```python
from build123d import *

# Parameters (mm, degrees)
SKETCH1_R           = 2.5
BOSS_EXTRUDE1_DEPTH = 4
SKETCH2_R           = 5
BOSS_EXTRUDE2_DEPTH = 0.75
M1_6_NUT_DEPTH      = 9.124038405
M1_6_NUT_DEPTH_BACK = 9.124038405
SKETCH5_W           = 6.5
SKETCH5_H           = 0.25
CUT_EXTRUDE1_DEPTH  = 9.124038405


with BuildPart() as part:
    # Sketch1 → Boss-Extrude1 (new, symmetric)
    with BuildSketch(Plane(origin=(0, 0, 0), x_dir=(0, 0, -1), z_dir=(1, 0, 0))):
        Circle(SKETCH1_R)
    extrude(amount=BOSS_EXTRUDE1_DEPTH, both=True)

    # Sketch2 → Boss-Extrude2 (add)
    with BuildSketch(Plane(origin=(4, 0, 0), x_dir=(0, 0, -1), z_dir=(1, 0, 0))):
        Circle(SKETCH2_R)
    boss_extrude2 = extrude(amount=-BOSS_EXTRUDE2_DEPTH)

    # Mirror1: Boss-Extrude2 across plane
    add(boss_extrude2.mirror(Plane(origin=(0, 0, 0), x_dir=(0, 0, 1), z_dir=(1, 0, 0))))

    # Sketch3 → M1.6 Nut (cut, two sides: drawn at the far end of the back side and taken through both)
    with BuildSketch(Plane(origin=(0, 0, 0), x_dir=(0, 0, -1), z_dir=(1, 0, 0)).offset(-M1_6_NUT_DEPTH_BACK)):
        Polygon((1.75, 0), (1.75, 1.010362971), (0.875, 1.515544457), (0, 2.020725942), (-0.875, 1.515544457), (-1.75, 1.010362971), (-1.75, 0), (-1.75, -1.010362971), (-0.875, -1.515544457), (0, -2.020725942), (0.875, -1.515544457), (1.75, -1.010362971), align=None)
    extrude(amount=M1_6_NUT_DEPTH + M1_6_NUT_DEPTH_BACK, mode=Mode.SUBTRACT)

    # Sketch5 → Cut-Extrude1 (cut, through all)
    with BuildSketch(Plane.XY):
        Rectangle(SKETCH5_W, SKETCH5_H)
    extrude(amount=CUT_EXTRUDE1_DEPTH, mode=Mode.SUBTRACT)


solid = part.part
```
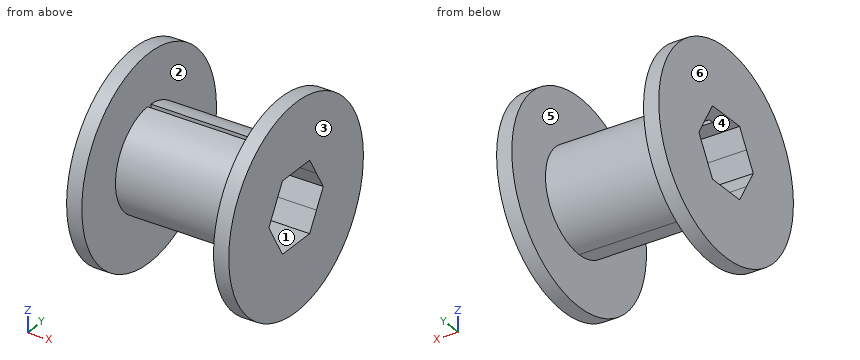
Part model, mm, in its own coordinate system. Face numbers are marked on the shaded views. A direction names the side the tool comes from. Round coordinates to 2 decimals unless told otherwise and drop trailing zeros. Write each loop counter-clockwise with the first axis right and the second up, starting at its lowest first coordinate (ties: lowest second). Pieces come first, ordered by that corner, then holes. Notation, with made-up numbers: (-9.5, -30) -> (39.5, -30) arc R15 cw to (39.5, -4) -> close; hole circle Ø2 at (49.25, 80). An arc over 180 degrees is marked (long way). Return JSON: item names as keys, results as strings. Group by question number.
Q1. Saw through at C-C on x = -1.75. Write the cut outline in (y, z) (3 decimals).
Q2. Which spindle directions (+Z, -Z, +X, -X, +Y, -Y) get a long thin tool onto all of the face, cutting with end or side? Do the marked faces 1, 2 and 3. Say none if no direction does.
Q3. Saw through at B-B on y = 2.75. Write the cut outline in (x, z).
Q4. Probe L1, parallel to X at y = -1.5, z = -3.75; L2, parallel to Y at x = -0.25, z = -0.5; L3, parallel to Y at x = -2.5, z = 1.5. List the from-to ranges inside material, lowest first. Write a range as [from, to].
Q5. Pin check, flat tips, straight feed: pin 1 (1.5 mm diameter, centred on x = 0, z = 0.5, fed in from -Y); pin 2 (2 mm diameter, centred on x = 1.5, z = 2.5, fed in from -Y); pin 3 (1 mm diameter, centred on x = -2.5, z = 0, fed in from +Y). Stop position of each tip, or through.
Q6. Saw through at D-D on z = 1.5. Write the cut outline in (x, y), plus the area to 3 significant figures.
Q7. Mould opens along X. For the marked faces 4, 5 and 6 say: pulls with the +X half, pulls with the -X half, needs draft (parallel to the pull), parting line crosses it, or undercut.
Q8. Saw through at A-A on z = -3. Write the cut outline in (x, y), plus the area to 3 significant figures.
Answer:
{
 "1": {"outline": "(-2.021, 0) -> (-1.01, 1.75) -> (-0.125, 1.75) -> (-0.125, 2.497) arc R2.5 ccw (long way) to (0.125, 2.497) -> (0.125, 1.75) -> (1.01, 1.75) -> (2.021, 0) -> (1.01, -1.75) -> (-1.01, -1.75) -> close"},
 "2": {"face 1": "+X, -X", "face 2": "none", "face 3": "+Z, -Z, +X, +Y, -Y"},
 "3": {"outline": "(-4, -4.18) -> (-3.25, -4.18) -> (-3.25, 4.18) -> (-4, 4.18) -> close; (3.25, -4.18) -> (4, -4.18) -> (4, 4.18) -> (3.25, 4.18) -> close"},
 "4": {"L1": "[-4, -3.25], [3.25, 4]", "L2": "[-2.45, -1.73], [1.73, 2.45]", "L3": "[-2, -1.15], [1.15, 2]"},
 "5": {"pin 1": "y = -2.5", "pin 2": "y = -2", "pin 3": "y = 2.5"},
 "6": {"outline": "(-4, -4.77) -> (-3.25, -4.77) -> (-3.25, -2) -> (3.25, -2) -> (3.25, -4.77) -> (4, -4.77) -> (4, -1.15) -> (-4, -1.15) -> close; (-4, 1.15) -> (4, 1.15) -> (4, 4.77) -> (3.25, 4.77) -> (3.25, 2) -> (-3.25, 2) -> (-3.25, 4.77) -> (-4, 4.77) -> close", "area": "21.8 mm2"},
 "7": {"face 4": "needs draft", "face 5": "undercut", "face 6": "pulls with the -X half"},
 "8": {"outline": "(-4, -4) -> (-3.25, -4) -> (-3.25, 4) -> (-4, 4) -> close; (3.25, -4) -> (4, -4) -> (4, 4) -> (3.25, 4) -> close", "area": "12.0 mm2"}
}
